from build123d import *

# Parameters (mm, degrees)
F0_R     = 12.7
F0_R_2   = 6.35
F1_DEPTH = 12.7
F2_DEPTH = 279.4
F5_DEPTH = 25.4
F7_DEPTH = 25.4


with BuildPart() as f1:
    # F0 (on Front) → F1 (new body)
    with BuildSketch(Plane.XZ):
        Circle(F0_R)
        Circle(F0_R_2, mode=Mode.SUBTRACT)
        Circle(F0_R_2)
    extrude(amount=-F1_DEPTH)

    # F0 (on Front) → F2 (join)
    with BuildSketch(Plane.XZ):
        Circle(F0_R)
        Circle(F0_R_2, mode=Mode.SUBTRACT)
    extrude(amount=-F2_DEPTH)

    # F4 (on Right) → F5 (cut)
    with BuildSketch(Plane.YZ):
        with BuildLine():
            ThreePointArc((18.25625, 0), (19.05, -0.79375), (19.84375, 0))
            ThreePointArc((19.84375, 0), (19.05, 0.79375), (18.25625, 0))
        make_face()
    extrude(amount=-F5_DEPTH, mode=Mode.SUBTRACT)

    # F6 (on Right) → F7 (cut)
    with BuildSketch(Plane.YZ):
        with BuildLine():
            ThreePointArc((248.44375, 0), (247.65, 0.79375), (246.85625, 0))
            Line((246.85625, 0), (247.65, 0))
            Line((247.65, 0), (248.44375, 0))
        make_face()
        with BuildLine():
            Line((247.65, 0), (246.85625, 0))
            ThreePointArc((246.85625, 0), (247.65, -0.79375), (248.44375, 0))
            Line((248.44375, 0), (247.65, 0))
        make_face()
    extrude(amount=-F7_DEPTH, mode=Mode.SUBTRACT)


solid = f1.part
Read the model definition and answer for the solid it produces. Units are mm, in the model's axes. A direction names the side the tool comes from. Round coordinates to 2 decimals unless told otherwise and drop trailing zeros. Write each loop counter-clockwise with the first axis right and the second up, starting at its lowest first coordinate (ties: lowest second). Pieces come first, ordered by that corner, then holes. Notation, with made-up numbers: (22, 33) - (35, 33) arc R13 ccw to (35, 58) - close; hole circle Ø8 at (73.25, 85). An arc over 180 degrees is marked (long way). One line per question, with ' | ' between items. Start each with the question number.
1. For a pull along Z with two mould halves and no side action, classify faces 1 (the face through (0, 12.7, 0)), 2 (the face through (-2.75, 137.74, -12.4)), 3 (the face through (3, 279.4, 6)) as +Z half, -Z half, draft (parallel to the pull), parting line (faces both ways), or undercut.
2. For faces 4 (the face through (-1.38, 144.18, -6.2)), 5 (the face through (0, 0, 0)), determine the directions among +Z, -Z, +X, -X, +Y, -Y from which every point of the face is accessible in a straight line to the end or side of a thin tool.
3. Section D-D (x = 9.75) is taken. Determine the outline of the cut face in (y, z), and give its area (3 significant figures).
4. Section C-C (z = 3.5) is taken. Determine the outline of the cut face in (x, y).
5. Find the intervals of material crossed by probe 1 along X at (y, z) = (178, 0); probe 2 along Y at (x, z) = (1.5, -2.25), in increasing order. Write a range as [from, to].
6. Each of these flat-tipped pins is pushed along its axis until it touches: pin 1 (6 mm diameter, centred on x = -6, y = 245.5, fed in from +Z); pin 2 (1 mm diameter, centred on x = 8.5, y = 70, fed in from -Z); pin 3 (1.4 mm diameter, centred on y = 247.65, z = 0, fed in from -X). Where does it stop, or does it pass through?
7. Section B-B (y = 132.5) is taken. Determine the outline of the cut face in (x, z).
8. Section A-A (x = -1.25) is taken. Determine the outline of the cut face in (y, z).
Filled in:
1) face 1: undercut | face 2: parting line | face 3: draft
2) face 4: +Y | face 5: +Z, -Z, +X, -X, -Y
3) outline: (0, -8.14) - (279.4, -8.14) - (279.4, 8.14) - (0, 8.14) - close | area: 4,550 mm²
4) outline: (-12.21, 0) - (12.21, 0) - (12.21, 279.4) - (5.3, 279.4) - (5.3, 12.7) - (-5.3, 12.7) - (-5.3, 279.4) - (-12.21, 279.4) - close
5) probe 1: [-12.7, -6.35], [6.35, 12.7] | probe 2: [0, 12.7]
6) pin 1: z = 12.34 | pin 2: z = -9.86 | pin 3: x = 6.31
7) outline: circle Ø25.4 at (0, 0); hole circle Ø12.7 at (0, 0)
8) outline: (0, -12.64) - (279.4, -12.64) - (279.4, -6.23) - (12.7, -6.23) - (12.7, 6.23) - (279.4, 6.23) - (279.4, 12.64) - (0, 12.64) - close
